```python
from build123d import *

# Parameters (mm, degrees)
SKETCH1_W                       = 45
SKETCH1_H                       = 200
BOSS_EXTRUDE1_DEPTH             = 1700
FILLET1_R                       = 4
F_6_0MM_DOWEL_SLOT1_D           = 6
F_6_0MM_DOWEL_SLOT1_DEPTH       = 128.197418143
F_6_0MM_DOWEL_SLOT1_CSINK_D     = 6.05
F_6_0MM_DOWEL_SLOT1_CSINK_ANGLE = 90
F_6_0MM_DOWEL_SLOT1_TIP         = 1.802581857
SKETCH17_R                      = 18
CUT_EXTRUDE8_DEPTH              = 30
F_6_0MM_DOWEL_SLOT3_D           = 6
F_6_0MM_DOWEL_SLOT3_DEPTH       = 63.197418143
F_6_0MM_DOWEL_SLOT3_CSINK_D     = 6.05
F_6_0MM_DOWEL_SLOT3_CSINK_ANGLE = 90
F_6_0MM_DOWEL_SLOT3_TIP         = 1.802581857
F_6_0MM_DOWEL_SLOT4_D           = 6
F_6_0MM_DOWEL_SLOT4_DEPTH       = 48.197418143
F_6_0MM_DOWEL_SLOT4_CSINK_D     = 6.05
F_6_0MM_DOWEL_SLOT4_CSINK_ANGLE = 90
F_6_0MM_DOWEL_SLOT4_TIP         = 1.802581857
SKETCH22_R                      = 18
CUT_EXTRUDE9_DEPTH              = 30
F_8_0MM_DOWEL_SLOT3_D           = 8
F_8_0MM_DOWEL_SLOT3_DEPTH       = 137.596557524
F_8_0MM_DOWEL_SLOT3_CSINK_D     = 8.05
F_8_0MM_DOWEL_SLOT3_CSINK_ANGLE = 90
F_8_0MM_DOWEL_SLOT3_TIP         = 2.403442476
F_6_0MM_DOWEL_SLOT8_D           = 6
F_6_0MM_DOWEL_SLOT8_DEPTH       = 28.197418143
F_6_0MM_DOWEL_SLOT8_CSINK_D     = 6.05
F_6_0MM_DOWEL_SLOT8_CSINK_ANGLE = 90
F_6_0MM_DOWEL_SLOT8_TIP         = 1.802581857


with BuildPart() as part:
    # Sketch1 → Boss-Extrude1 (new body)
    with BuildSketch(Plane.XY):
        with Locations((-8.688255411, 34.272684877)):
            Rectangle(SKETCH1_W, SKETCH1_H)
    extrude(amount=BOSS_EXTRUDE1_DEPTH)

    # Fillet1
    fillet1_edges = [part.edges().sort_by_distance(p)[0] for p in [
        (13.811744589, 134.272684877, 850),
        (13.811744589, -65.727315123, 850),
        (-31.188255411, -65.727315123, 850),
        (-31.188255411, 134.272684877, 850),
    ]]
    fillet(fillet1_edges, radius=FILLET1_R)

    # Ø6.0mm Dowel Slot1
    with Locations(Plane(origin=(495.936786729, -65.727315123, 442.277224535), x_dir=(0.6427592920058945, -7.13765947743485e-15, -0.7660682035824756), z_dir=(0.7660682035824756, -8.506969936751697e-15, 0.6427592920058945))):
        with Locations((-717.573535848, 40), (-343.837284168, -87.348590076), (-717.573535848, 100), (-645.06893427, -63.697919268), (-717.573535848, 160)):
            CounterSinkHole(F_6_0MM_DOWEL_SLOT1_D / 2, F_6_0MM_DOWEL_SLOT1_CSINK_D / 2, depth=F_6_0MM_DOWEL_SLOT1_DEPTH, counter_sink_angle=F_6_0MM_DOWEL_SLOT1_CSINK_ANGLE)
            with Locations((0, 0, -(F_6_0MM_DOWEL_SLOT1_DEPTH + F_6_0MM_DOWEL_SLOT1_TIP / 2))):  # 118° drill point
                Cone(0, F_6_0MM_DOWEL_SLOT1_D / 2, F_6_0MM_DOWEL_SLOT1_TIP, mode=Mode.SUBTRACT)

    # Sketch17 → Cut-Extrude8 (cut)
    with BuildSketch(Plane(origin=(13.811744589, 0, 0), x_dir=(0, 0, -1), z_dir=(1, 0, 0))):
        with Locations((-50, -25.727315123)):
            Circle(SKETCH17_R)
        with Locations((-50, 34.272684877)):
            Circle(SKETCH17_R)
        with Locations((-50, 91.272684877)):
            Circle(SKETCH17_R)
    extrude(amount=-CUT_EXTRUDE8_DEPTH, mode=Mode.SUBTRACT)

    # Ø6.0mm Dowel Slot3
    with Locations(Plane(origin=(-31.188255411, -65.727315123, 0), x_dir=(0, 0, 1), z_dir=(-1, 0, 0))):
        with Locations((872.5, 160), (872.5, 100), (872.5, 40)):
            CounterSinkHole(F_6_0MM_DOWEL_SLOT3_D / 2, F_6_0MM_DOWEL_SLOT3_CSINK_D / 2, depth=F_6_0MM_DOWEL_SLOT3_DEPTH, counter_sink_angle=F_6_0MM_DOWEL_SLOT3_CSINK_ANGLE)
            with Locations((0, 0, -(F_6_0MM_DOWEL_SLOT3_DEPTH + F_6_0MM_DOWEL_SLOT3_TIP / 2))):  # 118° drill point
                Cone(0, F_6_0MM_DOWEL_SLOT3_D / 2, F_6_0MM_DOWEL_SLOT3_TIP, mode=Mode.SUBTRACT)

    # Ø6.0mm Dowel Slot4
    with Locations(Plane(origin=(-31.188255411, -65.727315123, 1700), x_dir=(1, 0, 0), z_dir=(0, 0, 1))):
        with Locations((25, 160), (25, 40), (800, 160), (800, 40)):
            CounterSinkHole(F_6_0MM_DOWEL_SLOT4_D / 2, F_6_0MM_DOWEL_SLOT4_CSINK_D / 2, depth=F_6_0MM_DOWEL_SLOT4_DEPTH, counter_sink_angle=F_6_0MM_DOWEL_SLOT4_CSINK_ANGLE)
            with Locations((0, 0, -(F_6_0MM_DOWEL_SLOT4_DEPTH + F_6_0MM_DOWEL_SLOT4_TIP / 2))):  # 118° drill point
                Cone(0, F_6_0MM_DOWEL_SLOT4_D / 2, F_6_0MM_DOWEL_SLOT4_TIP, mode=Mode.SUBTRACT)

    # Sketch22 → Cut-Extrude9 (cut)
    with BuildSketch(Plane(origin=(13.811744589, -65.727315123, 0), x_dir=(0, 0, -1), z_dir=(1, 0, 0))):
        with Locations((-1650, 160)):
            Circle(SKETCH22_R)
        with Locations((-1650, 40)):
            Circle(SKETCH22_R)
    extrude(amount=-CUT_EXTRUDE9_DEPTH, mode=Mode.SUBTRACT)

    # Ø8.0mm Dowel Slot3
    with Locations(Plane(origin=(-31.188255411, -65.727315123, -90), x_dir=(-1, 0, 0), z_dir=(0, 0, -1))):
        with Locations((-22.5, 40), (-22.5, 100), (-22.5, 157)):
            CounterSinkHole(F_8_0MM_DOWEL_SLOT3_D / 2, F_8_0MM_DOWEL_SLOT3_CSINK_D / 2, depth=F_8_0MM_DOWEL_SLOT3_DEPTH, counter_sink_angle=F_8_0MM_DOWEL_SLOT3_CSINK_ANGLE)
            with Locations((0, 0, -(F_8_0MM_DOWEL_SLOT3_DEPTH + F_8_0MM_DOWEL_SLOT3_TIP / 2))):  # 118° drill point
                Cone(0, F_8_0MM_DOWEL_SLOT3_D / 2, F_8_0MM_DOWEL_SLOT3_TIP, mode=Mode.SUBTRACT)

    # Ø6.0mm Dowel Slot8
    with Locations(Plane(origin=(-31.188255411, 146.272684877, 0), x_dir=(1, 0, 0), z_dir=(0, 1, 0))):
        with Locations((22.5, 1726.5), (22.5, 1640.5), (802.5, 1726.5), (802.5, 1640.5), (22.5, -955.960621131), (22.5, -1636.5), (802.5, -1462.5), (802.5, -1636.5), (22.5, -1722.5), (802.5, -1722.5), (22.5, -1550.5), (802.5, -640.31), (120, -1722.5), (217.5, -1722.5), (315, -1722.5), (412.5, -1722.5), (510, -1722.5), (607.5, -1722.5), (705, -1722.5), (22.5, -861.25), (22.5, -883.75), (-22.496198074, -917.60220409), (802.5, -861.25), (802.5, -883.75), (847.496198074, -917.60220409), (802.5, -529.84), (22.5, -750.249617159), (-341.005231297, -650.318686522), (1166.005231297, -650.318686522), (-310.084924074, 22.5), (-310.084924074, 67.5), (22.5, 67.5), (22.5, 22.5), (802.5, 67.5), (802.5, 22.5), (1133.730020848, 67.5), (1133.730020848, 22.5), (1166.005231297, 740.318686522), (802.560751791, 973.75), (802.560751791, 951.25), (847.496198074, 1007.60220409), (-22.496198074, 1007.60220409), (22.560751791, 951.25), (-341.005231297, 740.318686522), (22.5, 1812.5), (802.5, 1812.5), (22.5, 1552.5), (802.5, 1552.5), (-102.162023695, -850.748960129), (-181.827849315, -783.895716167), (-261.493674936, -717.042472206), (927.162023695, -850.748960129), (1006.827849315, -783.895716167), (1086.493674936, -717.042472206), (1086.493674936, 807.042472206), (1006.827849315, 873.895716167), (927.162023695, 940.748960129), (-102.162023695, 940.748960129), (-181.827849315, 873.895716167), (-261.493674936, 807.042472206), (-199.224924074, 67.5), (-88.364924074, 67.5), (-199.224924074, 22.5), (-88.364924074, 22.5), (912.010020848, 67.5), (1022.870020848, 67.5), (912.010020848, 22.5), (1022.870020848, 22.5), (120, 67.5), (217.5, 67.5), (315, 67.5), (607.5, 67.5), (705, 67.5), (510, 67.5), (120, 22.5), (217.5, 22.5), (315, 22.5), (510, 22.5), (607.5, 22.5), (705, 22.5), (412.5, 22.5), (22.5, -750.78), (22.5, -640.31), (22.5, -529.84), (22.5, -419.37), (22.5, -308.9), (22.5, -198.43), (22.5, -87.96), (802.5, -750.78), (802.5, -419.37), (802.5, -308.9), (802.5, -198.43), (22.5, 177.97), (22.5, 288.44), (22.5, 398.91), (22.5, 509.38), (22.5, 619.85), (22.5, 730.32), (22.5, 840.79), (802.5, -87.96), (802.5, 177.97), (802.5, 288.44), (120.000330201, 1812.753749877), (217.5, 1812.5), (315, 1812.5), (412.5, 1812.5), (510, 1812.5), (607.5, 1812.5), (705, 1812.5), (120.060751791, 951.25), (217.560751791, 951.25), (315.060751791, 951.25), (412.560751791, 951.25), (510.060751791, 951.25), (607.560751791, 951.25), (705.060751791, 951.25), (656.310751791, 973.75), (558.810751791, 973.75), (461.310751791, 973.75), (363.810751791, 973.75), (266.310751791, 973.75), (168.810751791, 973.75), (120, -861.25), (217.5, -861.25), (315, -861.25), (412.5, -861.25), (510, -861.25), (607.5, -861.25), (705, -861.25), (656.25, -883.75), (558.75, -883.75), (461.25, -883.75), (168.75, -883.75), (266.25, -883.75), (363.75, -883.75), (802.560751791, -955.960621131), (412.5, 67.5), (802.5, 730.32), (802.560751791, 840.79), (802.5, 398.91), (802.5, 509.38), (802.5, 619.85), (-360.000025903, 699.425529794), (-360.000025903, -609.521258848), (-360.000025903, 598.725529794), (-360.000025903, 498.025529794), (-360.000025903, 397.325529794), (-360.000025903, 296.625529794), (-360.000025903, 195.925529794), (-360.000025903, 95.225529794), (-360.000025903, -5.474470206), (-360.000025903, -106.174470206), (-360.000025903, -206.874470206), (-360.000025903, -307.574470206), (-360.000025903, -408.274470206), (-360.000025903, -508.974470206), (1185.00101945, 699.425529452), (1185.000941829, 598.725529794), (1185.000864209, 498.025529794), (1185.000708968, 296.625529794), (1185.000631348, 195.925529794), (1185.000553727, 95.225529794), (1185.000476107, -5.474470206), (1185.000398486, -106.174470206), (1185.000320866, -206.874470206), (1185.000165625, -408.274470206), (1185.000088004, -508.974470206), (1185.000786589, 397.325529794), (22.560751791, 1016.385842825), (802.560751791, 1016.385842825), (802.560751791, -1550.5), (22.560751791, 973.75), (802.560751791, -363.966698641)):
            CounterSinkHole(F_6_0MM_DOWEL_SLOT8_D / 2, F_6_0MM_DOWEL_SLOT8_CSINK_D / 2, depth=F_6_0MM_DOWEL_SLOT8_DEPTH, counter_sink_angle=F_6_0MM_DOWEL_SLOT8_CSINK_ANGLE)
            with Locations((0, 0, -(F_6_0MM_DOWEL_SLOT8_DEPTH + F_6_0MM_DOWEL_SLOT8_TIP / 2))):  # 118° drill point
                Cone(0, F_6_0MM_DOWEL_SLOT8_D / 2, F_6_0MM_DOWEL_SLOT8_TIP, mode=Mode.SUBTRACT)


solid = part.part
```
Can you work these out from the model? Positions are in its coordinate system, mm. A direction names the side the tool comes from. Round coordinates to 2 decimals unless told otherwise and drop trailing zeros. Loops run counter-clockwise (first coordinate to the right, second up) from the corner with the lowest first, then second, coordinate; pieces in that order, holes last. Notation, with made-up numbers: M 10,-31 L 39,-31 A31 cw 39,7 Z; hole C 11,-38 d8. An arc over 180 degrees is marked long. Answer as a JSON object with one key per item and string values. Group by question number.
Q1. On a 3-axis mill with a long thin cutter (end or side, diameter ignored), from which of +Z, -Z, +X, -X, +Y, -Y can I reach the whole of each face in a straight line? I mean faces 1 (the flat face through (-16.188, 92, 50)), 2 (the cylindrical face through (-7.14, 94.4, 952.96)). Say none if no direction works.
Q2. Will this pin go through, and if not, where does the flat tip stop? pin 1 (3.5 mm diameter, centred on x = -6.19, y = -25.73, fed in from +Z).
Q3. Imagine slicing it at A-A, the plane z = 50. Please give me the cut outline in (x, y).
Q4. Please list where these lines run through material, in increasing order: L1, parallel to Y at x = -6, z = 1650; L2, parallel to Y at x = -19, z = 872; L3, parallel to X at y = 122.75, z = 87.96.
Q5. We'd pull the mould along Y, two halves only. Please class faces 3 (the flat face through (-9, 36, 1700)), 4 (the cylindrical face through (-0.98, 99.68, 1632.83)), 5 (the flat face through (-9, -65.727, 838)), 6 (the flat face through (-9, 134.273, 838)): +Y half, -Y half, draft (parallel to the pull), parting line (faces both ways), or undercut.
Findings:
{
 "1": {"face 1": "+X", "face 2": "none"},
 "2": {"pin 1": "stops at z = 1632.09"},
 "3": {"outline": "M -31.19,-61.73 A4 ccw -27.19,-65.73 L 9.81,-65.73 A4 ccw 13.81,-61.73 L 13.81,-43.73 L -16.19,-43.73 L -16.19,-7.73 L 13.81,-7.73 L 13.81,16.27 L -16.19,16.27 L -16.19,52.27 L 13.81,52.27 L 13.81,73.27 L -16.19,73.27 L -16.19,109.27 L 13.81,109.27 L 13.81,130.27 A4 ccw 9.81,134.27 L -27.19,134.27 A4 ccw -31.19,130.27 Z"},
 "4": {"L1": "y = -65.73 to -43.73, -7.73 to 76.27, 112.27 to 134.27", "L2": "y = -65.73 to -28.69, -22.77 to 31.31, 37.23 to 91.31, 97.23 to 134.27", "L3": "x = -31.19 to -11.69, -5.69 to 13.81"},
 "5": {"face 3": "draft", "face 4": "undercut", "face 5": "-Y half", "face 6": "+Y half"}
}
